```python
from build123d import *

# Parameters (mm, degrees)
BOSS_EXTRUDE1_DEPTH = 5
CUT_EXTRUDE1_DEPTH  = 5
CHAMFER1_SIZE       = 3


with BuildPart() as part:
    # Sketch1 → Boss-Extrude1 (new body)
    with BuildSketch(Plane(origin=(0, 0, 0), x_dir=(1, 0, 0), z_dir=(0, 1, 0))):
        with BuildLine():
            Line((0, -4), (0, -2))
            ThreePointArc((0, -2), (-1.414213562, 1.414213562), (2, 0))
            Line((2, 0), (3, 0))
            Line((3, 0), (3, -3.760972677))
            Line((3, -3.760972677), (4.998650065, -3.760972677))
            Line((4.998650065, -3.760972677), (5.005216321, -3.757452983))
            Line((5.005216321, -3.757452983), (5.005216321, 4))
            Line((5.005216321, 4), (0, 4))
            ThreePointArc((0, 4), (-4, 0), (0, -4))
        make_face()
    extrude(amount=BOSS_EXTRUDE1_DEPTH)

    # Sketch2 → Cut-Extrude1 (cut)
    with BuildSketch(Plane(origin=(0, 0, 0), x_dir=(0, 0, -1), z_dir=(1, 0, 0))):
        Polygon((4, 5), (0, 5), (0, 4.983533527), (-4, 4.983533527), (-4, 1.983533527), (0, 1.983533527), (0, 4), (4, 4), align=None)
    extrude(amount=-CUT_EXTRUDE1_DEPTH, mode=Mode.SUBTRACT)


with BuildPart() as cut_extrude1_kept_piece:
    # of the separate pieces the step leaves, the one the design keeps (cut_extrude1_pieces_kept)
    add(part.part.solids().sort_by_distance((0, 0, 4))[0])

    # Chamfer1
    chamfer1_edges = [cut_extrude1_kept_piece.edges().sort_by_distance(p)[0] for p in [
        (3.999325033, 5, 3.760972677),
    ]]
    chamfer(chamfer1_edges, length=CHAMFER1_SIZE)


solid = cut_extrude1_kept_piece.part
```
Verification items for the finished model (mm, model axes). A direction names the side the tool comes from. Give positions to 0.01 mm unless a question says otherwise; leave off trailing zeros. Order: outer loops, then holes, each group sorted by start corner. A loop starts at its lowest first (then second) coordinate and runs counter-clockwise, first axis right, second up. Notation, with made-up numbers: M 33,66.25 L 88,66.25 A20 ccw 88,80.25 Z; hole C -21,-38 d11. An arc over 180 degrees is marked long. Answer in a Markdown table with one row per item. Add a question column.
Item 1: Tool access check on faces 1 (the flat face through (-2, 4, -2)), 2 (the flat face through (2.5, 2.5, 0)), 3 (the flat face through (4, 1, 3.761)), 4 (the flat face through (-2, 1.984, 2)), 5 (the flat face through (3, 5, -2)). Record the directions out of +Z, -Z, +X, -X, +Y, -Y that give a thin tool (end or side, any length) a straight path to the whole face; none if there is none.
Item 2: Section check D-D, the plane z = -2.75. Enter the section's corners in (x, y), and give its area (3 significant figures).
Item 3: Scan lines: probe 1 along Z at (x, y) = (0, 2.7); probe 2 along Y at (x, z) = (3.75, 2); probe 3 along X at (y, z) = (3.85, -1). Record each from-to range of solid material in increasing order. Write a range as from..to.
Item 4: Gauge pin test, flat ends, axial feed: pin 1 (1.5 mm diameter, centred on x = 0, z = 1.5, fed in from +Y); pin 2 (1.1 mm diameter, centred on x = 2.5, y = 2, fed in from +Z); pin 3 (1.9 mm diameter, centred on y = 3.5, z = 2, fed in from -X). Record the tip position at first contact, or that the pin passes through.
Item 5: Section check A-A, the plane z = 1. Enter the section's corners in (x, y).
Item 6: Section check C-C, the plane x = 2.25. Enter the section's corners in (y, z).
Item 7: Mould release check, pull along Z, two halves, no side actions. Record for faces 6 (the flat face through (3, 2, -4)), 7 (the flat face through (5.005, 2, 0)), 8 (the cylindrical face through (-3.73, 1.53, -1.45)), 9 (the cylindrical face through (-0.581, 1.909, -1.914)): released by +Z, released by -Z, zero draft, split by the parting line, or undercut.
Filled sheet:
| question | item | result |
|---|---|---|
| 1 | face 1 | +Z, -Z, -X, +Y |
| 1 | face 2 | +Z, +Y, -Y |
| 1 | face 3 | +Z, +X, +Y, -Y |
| 1 | face 4 | +Z, -X, +Y |
| 1 | face 5 | +Z, -Z, +X, -X, +Y |
| 2 | outline | M -2.9,0 L 5.01,0 L 5.01,5 L 0,5 L 0,4 L -2.9,4 Z |
| 2 | area | 36.6 mm^2 |
| 3 | probe 1 | z = -4..-2 |
| 3 | probe 2 | y = 0..3.76 |
| 3 | probe 3 | x = -3.87..-1.73, 1.73..5.01 |
| 4 | pin 1 | stops at y = 1.98 |
| 4 | pin 2 | stops at z = 3.76 |
| 4 | pin 3 | stops at x = 3 |
| 5 | outline | M -3.87,0 L -1.73,0 L -1.73,1.98 L -3.87,1.98 Z; M 3,0 L 5.01,0 L 5.01,4.76 L 3,4.76 Z |
| 6 | outline | M 0,-4 L 5,-4 L 5,0 L 0,0 Z |
| 7 | face 6 | released by -Z |
| 7 | face 7 | zero draft |
| 7 | face 8 | split by the parting line |
| 7 | face 9 | undercut |
